from build123d import *

# Parameters (mm, degrees)
ESQUISSE1_W                  = 720
ESQUISSE1_H                  = 25
BOSS_EXTRU_1_DEPTH           = 25
BOSS_EXTRU_1_2_DEPTH         = 25
ENL_V_MAT_EXTRU_1_DEPTH      = 25
ENL_V_MAT_EXTRU_1_DEPTH_BACK = 100
ESQUISSE2_R                  = 4
ESQUISSE3_W                  = 25
ESQUISSE3_H                  = 25
BOSS_EXTRU_2_DEPTH           = 68
ESQUISSE4_W                  = 600
ESQUISSE4_H                  = 25
BOSS_EXTRU_3_DEPTH           = 25
ESQUISSE5_R                  = 2.75
ENL_V_MAT_EXTRU_2_DEPTH      = 25
ESQUISSE6_W                  = 25
ESQUISSE6_H                  = 1100
BOSS_EXTRU_4_DEPTH           = 25
ESQUISSE7_W                  = 25
ESQUISSE7_H                  = 25
BOSS_EXTRU_5_DEPTH           = 50
ESQUISSE8_W                  = 25
ESQUISSE8_H                  = 950
BOSS_EXTRU_6_DEPTH           = 25
ESQUISSE9_R                  = 2.75
ENL_V_MAT_EXTRU_3_DEPTH      = 25


with BuildPart() as part:
    # Esquisse1 → Boss.-Extru.1 (new body)
    with BuildSketch(Plane.XY):
        with Locations((360, 12.5)):
            Rectangle(ESQUISSE1_W, ESQUISSE1_H)
    extrude(amount=BOSS_EXTRU_1_DEPTH)


with BuildPart() as body_2:
    # Esquisse1 → Boss.-Extru.1 2 (new body)
    with BuildSketch(Plane.XY):
        with Locations((360, -1112.5)):
            Rectangle(ESQUISSE1_W, ESQUISSE1_H)
    extrude(amount=BOSS_EXTRU_1_2_DEPTH)


with BuildPart() as enl_v_mat_extru_1_tool:
    # Esquisse2 → Enlèv. mat.-Extru.1 (new, two sides: drawn at the far end of the back side and taken through both)
    with BuildSketch(Plane.XY.offset(25).offset(-ENL_V_MAT_EXTRU_1_DEPTH_BACK)):
        with Locations(Location((10, 12.5, 0), (0, 0, 180))):
            Circle(ESQUISSE2_R)
        with Locations(Location((710, 12.5, 0), (0, 0, 180))):
            Circle(ESQUISSE2_R)
        with Locations(Location((710, -1112.5, 0), (0, 0, 180))):
            Circle(ESQUISSE2_R)
        with Locations(Location((10, -1112.5, 0), (0, 0, 180))):
            Circle(ESQUISSE2_R)
    extrude(amount=ENL_V_MAT_EXTRU_1_DEPTH + ENL_V_MAT_EXTRU_1_DEPTH_BACK)


with BuildPart() as part_1:
    add(part.part)

    # Enlèv. mat.-Extru.1: cut by enl_v_mat_extru_1_tool
    add(enl_v_mat_extru_1_tool.part, mode=Mode.SUBTRACT)



with BuildPart() as body_2_1:
    add(body_2.part)

    # Enlèv. mat.-Extru.1: cut by enl_v_mat_extru_1_tool
    add(enl_v_mat_extru_1_tool.part, mode=Mode.SUBTRACT)


with BuildPart() as part_2:
    add(part_1.part)

    add(body_2_1.part)  # Boss.-Extru.2 merges body 2
    # Esquisse3 → Boss.-Extru.2 (add)
    with BuildSketch(Plane.XY.offset(25)):
        with Locations((72.5, 12.5)):
            Rectangle(ESQUISSE3_W, ESQUISSE3_H)
        with Locations((647.5, 12.5)):
            Rectangle(ESQUISSE3_W, ESQUISSE3_H)
        with Locations((72.5, -1112.5)):
            Rectangle(ESQUISSE3_W, ESQUISSE3_H)
        with Locations((647.5, -1112.5)):
            Rectangle(ESQUISSE3_W, ESQUISSE3_H)
    extrude(amount=BOSS_EXTRU_2_DEPTH)

    # Esquisse4 → Boss.-Extru.3 (add)
    with BuildSketch(Plane.XY.offset(93)):
        with Locations((360, 12.5)):
            Rectangle(ESQUISSE4_W, ESQUISSE4_H)
        with Locations((360, -1112.5)):
            Rectangle(ESQUISSE4_W, ESQUISSE4_H)
    extrude(amount=BOSS_EXTRU_3_DEPTH)

    # Esquisse5 → Enlèv. mat.-Extru.2 (cut)
    with BuildSketch(Plane.XY.offset(118)):
        with Locations((120, 12.5)):
            Circle(ESQUISSE5_R)
        with Locations((600, 12.5)):
            Circle(ESQUISSE5_R)
        with Locations((600, -1112.5)):
            Circle(ESQUISSE5_R)
        with Locations((120, -1112.5)):
            Circle(ESQUISSE5_R)
    extrude(amount=-ENL_V_MAT_EXTRU_2_DEPTH, mode=Mode.SUBTRACT)

    # Esquisse6 → Boss.-Extru.4 (add)
    with BuildSketch(Plane(origin=(0, 0, 0), x_dir=(-1, 0, 0), z_dir=(0, 0, -1))):
        with Locations((-675, -550)):
            Rectangle(ESQUISSE6_W, ESQUISSE6_H)
        with Locations((-45, -550)):
            Rectangle(ESQUISSE6_W, ESQUISSE6_H)
    extrude(amount=-BOSS_EXTRU_4_DEPTH)

    # Esquisse7 → Boss.-Extru.5 (add)
    with BuildSketch(Plane.XY.offset(25)):
        with Locations((45, -1012.5)):
            Rectangle(ESQUISSE7_W, ESQUISSE7_H)
        with Locations((45, -87.5)):
            Rectangle(ESQUISSE7_W, ESQUISSE7_H)
        with Locations((675, -87.5)):
            Rectangle(ESQUISSE7_W, ESQUISSE7_H)
        with Locations((675, -1012.5)):
            Rectangle(ESQUISSE7_W, ESQUISSE7_H)
    extrude(amount=BOSS_EXTRU_5_DEPTH)

    # Esquisse8 → Boss.-Extru.6 (add)
    with BuildSketch(Plane.XY.offset(75)):
        with Locations((675, -550)):
            Rectangle(ESQUISSE8_W, ESQUISSE8_H)
        with Locations((45, -550)):
            Rectangle(ESQUISSE8_W, ESQUISSE8_H)
    extrude(amount=BOSS_EXTRU_6_DEPTH)

    # Esquisse9 → Enlèv. mat.-Extru.3 (cut)
    with BuildSketch(Plane.XY.offset(100)):
        with Locations((675, -910)):
            Circle(ESQUISSE9_R)
        with Locations((45, -910)):
            Circle(ESQUISSE9_R)
        with Locations((675, -190)):
            Circle(ESQUISSE9_R)
        with Locations((45, -190)):
            Circle(ESQUISSE9_R)
    extrude(amount=-ENL_V_MAT_EXTRU_3_DEPTH, mode=Mode.SUBTRACT)


solid = part_2.part
The model under review builds one solid part; all positions refer to its coordinate system, in mm. A direction names the side the tool comes from. Round coordinates to 2 decimals unless told otherwise and drop trailing zeros. Write each loop counter-clockwise with the first axis right and the second up, starting at its lowest first coordinate (ties: lowest second). Pieces come first, ordered by that corner, then holes. Notation, with made-up numbers: M -23,-33 L 2,-33 A29 cw 2,-9 Z; hole C 30.5,77.25 d5. An arc over 180 degrees is marked long. Answer as CSV lines item,"result". Start each with the question number.
Q1. Wall thickness on line 1 along X through (y, z) = (-1112.5, 99.75); line 2 along Y through (x, z) = (675, 94); line 3 along Y through (x, z) = (600, 104): over which ranges is each line inside the solid? List them lowest first.
Q2. The part is to be moulded in two halves that separate along X. For faces 1 (the face through (720, -1113, 12)), 2 (the face through (675, -1025, 62)), 3 (the face through (356, -1100, 98)), say which applies: +X half, -X half, draft (parallel to the pull), parting line (faces both ways), or undercut.
Q3. Consider section B-B, the plane y = -114. Give the boundary of the cut face in (x, z).
Q4. Tool access review of faces 4 (the face through (45, -1025, 62)), 5 (the face through (676, -1085, 25)), 6 (the face through (675, -544, 25)): name each direction out of +Z, -Z, +X, -X, +Y, -Y from which nothing blocks a thin tool from reaching the whole face with its end or side.
Q5. Consider section C-C, the plane z = 45. State how many separate pieces and enclosed holes the cut face has, then the cut area to 3 significant figures.
Q6. Consider section A-A, the plane x = 177.5. Give the boundary of the cut face in (y, z), then the cut area to 3 significant figures.
Q7. Clearance check with flat-ended pins moving along their axes: P1, Ø10, axis at y = -891, z = 82.5, coming from the +X side; P2, Ø5, axis at x = 675, y = -910, coming from the +Z side; P3, Ø6, axis at y = -445, z = 25.5, coming from the -X side. State where each tip first meets the part, or that it passes through.
Result set:
1,line 1,"x = 60 to 117.25, 122.75 to 597.25, 602.75 to 660"
1,line 2,"y = -1025 to -912.75, -907.25 to -192.75, -187.25 to -75"
1,line 3,"y = -1125 to -1115.25, -1109.75 to -1100, 0 to 9.75, 15.25 to 25"
2,face 1,"+X half"
2,face 2,"draft"
2,face 3,"undercut"
3,outline,"M 32.5,0 L 57.5,0 L 57.5,25 L 32.5,25 Z; M 32.5,75 L 57.5,75 L 57.5,100 L 32.5,100 Z; M 662.5,0 L 687.5,0 L 687.5,25 L 662.5,25 Z; M 662.5,75 L 687.5,75 L 687.5,100 L 662.5,100 Z"
4,face 4,"+Z, +X, -X, -Y"
4,face 5,"+Z, +X, -Y"
4,face 6,"+X, -X"
5,separate pieces,"8"
5,enclosed holes,"0"
5,area,"5,000 mm²"
6,outline,"M -1125,0 L -1100,0 L -1100,25 L -1125,25 Z; M -1125,93 L -1100,93 L -1100,118 L -1125,118 Z; M 0,0 L 25,0 L 25,25 L 0,25 Z; M 0,93 L 25,93 L 25,118 L 0,118 Z"
6,area,"2,500 mm²"
7,P1,"stops at x = 687.5"
7,P2,"stops at z = 25"
7,P3,"stops at x = 32.5"
